Model file for the job. Use its own axes, mm. Coordinates: 2 decimals unless noted, no trailing zeros. Loops run counter-clockwise (first coordinate to the right, second up) from the corner with the lowest first, then second, coordinate; pieces in that order, holes last. Notation, with made-up numbers: (22.25, 20.5) -> (38.25, 20.5) arc R10 cw to (38.25, 35.5) -> close; hole circle Ø10 at (80.25, 63). An arc over 180 degrees is marked (long way). Use one line per item in the form item = value.
```python
from build123d import *

# Parameters (mm, degrees)
F1_DEPTH = 2.2


with BuildPart() as f1:
    # F0 (on Top) → F1 (new body, symmetric)
    with BuildSketch(Plane.XY):
        with BuildLine():
            ThreePointArc((-2.3937715127, -0.8788389756), (0, -2.55), (2.3937715127, -0.8788389756))
            Line((2.3937715127, -0.8788389756), (1.2767701653, -0.8788389756))
            ThreePointArc((1.2767701653, -0.8788389756), (0, -1.55), (-1.2767701653, -0.8788389756))
            Line((-1.2767701653, -0.8788389756), (-2.3937715127, -0.8788389756))
        make_face()
        with BuildLine():
            Line((1.2767701653, 0.8788389756), (2.3937715127, 0.8788389756))
            ThreePointArc((2.3937715127, 0.8788389756), (0, 2.55), (-2.3937715127, 0.8788389756))
            Line((-2.3937715127, 0.8788389756), (-1.2767701653, 0.8788389756))
            ThreePointArc((-1.2767701653, 0.8788389756), (0, 1.55), (1.2767701653, 0.8788389756))
        make_face()
        with BuildLine():
            ThreePointArc((2.3937715127, -0.8788389756), (2.5106390977, -0.4463085494), (2.55, 0))
            ThreePointArc((2.55, 0), (2.5106390977, 0.4463085494), (2.3937715127, 0.8788389756))
            Line((2.3937715127, 0.8788389756), (1.2767701653, 0.8788389756))
            ThreePointArc((1.2767701653, 0.8788389756), (1.4801171839, 0.4601664067), (1.55, 0))
            ThreePointArc((1.55, 0), (1.4801171839, -0.4601664067), (1.2767701653, -0.8788389756))
            Line((1.2767701653, -0.8788389756), (2.3937715127, -0.8788389756))
        make_face()
    extrude(amount=F1_DEPTH, both=True)


solid = f1.part
```
Q1. Band-saw the part on C-C, the plane x = 1.2. Write the cut outline in (y, z), and give its area (3 significant figures).
Result:
outline = (-2.25, -2.2) -> (-0.98, -2.2) -> (-0.98, 2.2) -> (-2.25, 2.2) -> close; (0.98, -2.2) -> (2.25, -2.2) -> (2.25, 2.2) -> (0.98, 2.2) -> close
area = 11.2 mm2
Q2. Band-saw the part on B-B, the plane z = 1.5. Write the cut outline in (x, y).
Result:
outline = (-2.39, -0.88) arc R2.55 ccw (long way) to (-2.39, 0.88) -> (-1.28, 0.88) arc R1.55 cw (long way) to (-1.28, -0.88) -> close
Q3. Band-saw the part on D-D, the plane y = 0.6. Write the cut outline in (x, z), and give its area (3 significant figures).
Result:
outline = (1.43, -2.2) -> (2.48, -2.2) -> (2.48, 2.2) -> (1.43, 2.2) -> close
area = 4.62 mm2
Q4. Mould opens along Y. For faces 1 (the face through (2, 0, -2.2)), 2 (the face through (-2, -0.879, 0)), 3 (the face through (2.55, -0.1, 0.03)) say: released by +Y, released by -Y, zero draft, split by the parting line, or undercut.
Result:
face_1 = zero draft
face_2 = undercut
face_3 = split by the parting line
Q5. Band-saw the part on A-A, the plane x = 0. Write the cut outline in (y, z), and give its area (3 significant figures).
Result:
outline = (-2.55, -2.2) -> (-1.55, -2.2) -> (-1.55, 2.2) -> (-2.55, 2.2) -> close; (1.55, -2.2) -> (2.55, -2.2) -> (2.55, 2.2) -> (1.55, 2.2) -> close
area = 8.80 mm2
Q6. Wall check: line 1 along X through (y, z) = (-1.25, 0.35); line 2 along X through (y, z) = (1.2, 1.05); line 3 along Y through (x, z) = (-0.15, 0.25). Give the ranges that are in metal, low to high.
Result:
line_1 = -2.22 to -0.92, 0.92 to 2.22
line_2 = -2.25 to -0.98, 0.98 to 2.25
line_3 = -2.55 to -1.54, 1.54 to 2.55
Q7. Pin check, flat tips, straight feed: pin 1 Ø1.2 at (x, z) = (-2, 0.5) entering from +Y; pin 2 Ø1 at (x, z) = (2, 0) entering from -Y. Stop position of each tip, or through.
Result:
pin_1 = 2.13
pin_2 = -2.06
